Verification items for the finished model (mm, model axes). A direction names the side the tool comes from. Coordinates: 2 decimals unless noted, no trailing zeros. Order: outer loops, then holes, each group sorted by start corner. A loop starts at its lowest first (then second) coordinate and runs counter-clockwise, first axis right, second up. Notation, with made-up numbers: (-33, -2.5) -> (5, -2.5) arc R17 cw to (5, 7.5) -> close; hole circle Ø5 at (86.25, -39). An arc over 180 degrees is marked (long way). Use CSV: the item, a comma, the result in double quotes. Start each with the question number.
1) Release check for a two-part mould opening along Y. For faces 3 (the flat face through (0, 1, 0)), 4 (the cylindrical face through (4.77, -36, 4.93)), 5 (the flat face through (0, 38, 10)), 6 (the cylindrical face through (-9.572, -57.282, 2.346)) record: released by +Y, released by -Y, zero draft, split by the parting line, or undercut.
2) Tool access check on faces 1 (the cylindrical face through (4.77, 39, 4.93)), 2 (the cylindrical face through (9.572, 57.282, 2.346)). Record the directions out of +Z, -Z, +X, -X, +Y, -Y that give a thin tool (end or side, any length) a straight path to the whole face; none if there is none.
3) Scan lines: line 1 along X through (y, z) = (37.5, 3); line 2 along Z through (x, y) = (6.3, -37.5); line 3 along Y through (x, z) = (-6.75, 6). Record each from-to range of solid material in increasing order.
4) Sectioned sample at A-A on z = 13.5. Record the boundary of the cut face in (x, y).
5) Go/stop test with flat-tipped pins: pin 1 (2.5 mm diameter, centred on y = -37.5, z = 6, fed in from +X); pin 2 (10 mm diameter, centred on x = 6.5, y = 59.5, fed in from -Z); pin 3 (3 mm diameter, centred on x = 2, y = -38, fed in from -Z); pin 4 (1.8 mm diameter, centred on y = 37.5, z = 6, fed in from -X). Record where each tip stops, or that it passes through.
from build123d import *

# Parameters (mm, degrees)
F0_R     = 5
F1_DEPTH = 18
F2_DEPTH = 10
F4_DEPTH = 20.001
F5_R     = 1.5
F6_R     = 3
F7_R     = 1
F8_DEPTH = 20.001


with BuildPart() as f1:
    # F0 (on Top) → F1 (new body)
    with BuildSketch(Plane.XY):
        with BuildLine():
            ThreePointArc((0, -75), (7.071068, -72.071068), (10, -65))
            Line((10, -65), (10, 65))
            ThreePointArc((10, 65), (7.071068, 72.071068), (0, 75))
            ThreePointArc((0, 75), (-7.071068, 72.071068), (-10, 65))
            Line((-10, 65), (-10, -65))
            ThreePointArc((-10, -65), (-7.071068, -72.071068), (0, -75))
        make_face()
        with Locations((0, -37.5)):
            Circle(F0_R, mode=Mode.SUBTRACT)
        with Locations((0, 37.5)):
            Circle(F0_R, mode=Mode.SUBTRACT)
        with Locations((0, -37.5)):
            Circle(F0_R)
        with Locations((0, 37.5)):
            Circle(F0_R)
    extrude(amount=F1_DEPTH)

    # F0 (on Top) → F2 (cut)
    with BuildSketch(Plane.XY):
        with Locations((0, -37.5)):
            Circle(F0_R)
        with Locations((0, 37.5)):
            Circle(F0_R)
    extrude(amount=F2_DEPTH, mode=Mode.SUBTRACT)

    # F3 (on face) → F4 (cut, through all)
    with BuildSketch(Plane.YZ.offset(10)):
        Polygon((-65, 0), (-65, 3.872983), (-88.729833, 10), (-88.729833, 0), align=None)
        Polygon((-65, 0), (-50, 0), (-65, 3.872983), align=None)
        Polygon((65, 3.872983), (65, 0), (88.729833, 0), (88.729833, 10), align=None)
        Polygon((65, 3.872983), (50, 0), (65, 0), align=None)
    extrude(amount=-F4_DEPTH, mode=Mode.SUBTRACT)

    # F5
    f5_edges = [f1.edges().sort_by_distance(p)[0] for p in [
        (10, -57.5, 1.936492),
        (10, 57.5, 1.936492),
        (10, 0, 0),
        (-10, 0, 0),
    ]]
    fillet(f5_edges, radius=F5_R)

    # F6
    f6_edges = [f1.edges().sort_by_distance(p)[0] for p in [
        (-10, 0, 18),
    ]]
    fillet(f6_edges, radius=F6_R)

    # F7 (on face) → F8 (cut, through all)
    with BuildSketch(Plane.YZ.offset(10)):
        with Locations((-37.5, 6)):
            Circle(F7_R)
        with Locations((37.5, 6)):
            Circle(F7_R)
    extrude(amount=-F8_DEPTH, mode=Mode.SUBTRACT)


solid = f1.part
Answers follow:
1,face 3,"zero draft"
1,face 4,"undercut"
1,face 5,"undercut"
1,face 6,"released by -Y"
2,face 1,"-Z"
2,face 2,"-Z, +X, +Y"
3,line 1,"x = -10 to -5, 5 to 10"
3,line 2,"z = 0 to 5, 7 to 18"
3,line 3,"y = -71.88 to -38.5, -36.5 to 36.5, 38.5 to 71.88"
4,outline,"(-10, -65) arc R10 ccw to (0, -75) arc R10 ccw to (10, -65) -> (10, 65) arc R10 ccw to (0, 75) arc R10 ccw to (-10, 65) -> close"
5,pin 1,"stops at x = 10"
5,pin 2,"stops at z = 1.16"
5,pin 3,"stops at z = 10"
5,pin 4,"passes through"
